Model file for the job. Use its own axes, mm. A direction names the side the tool comes from. Coordinates: 2 decimals unless noted, no trailing zeros. Order: outer loops, then holes, each group sorted by start corner. A loop starts at its lowest first (then second) coordinate and runs counter-clockwise, first axis right, second up. Notation, with made-up numbers: M 88.5,62 L 106.5,62 A29 ccw 106.5,89 Z; hole C 61.5,-38 d1. An arc over 180 degrees is marked long. Return JSON: item names as keys, results as strings.
```python
from build123d import *

# Parameters (mm, degrees)
F0_W     = 89
F0_H     = 23.8
F1_DEPTH = 3
F2_W     = 12
F2_H     = 6
F3_W     = 12
F3_H     = 6
F4_DEPTH = 9
F5_R     = 1.5
F6_DEPTH = 89.001
F7_R     = 1.5
F8_R     = 1.5
F9_DEPTH = 15


with BuildPart() as f1:
    # F0 (on Top) → F1 (new body)
    with BuildSketch(Plane.XY):
        Rectangle(F0_W, F0_H)
    extrude(amount=F1_DEPTH)

    # F2 (on face) + F3 (on face) → F4 (join)
    with BuildSketch(Plane.XY.offset(3)):
        with Locations((38.5, 8.9)):
            Rectangle(F2_W, F2_H)
    with BuildSketch(Plane.XY.offset(3)):
        with Locations((-38.5, 8.9)):
            Rectangle(F3_W, F3_H)
    extrude(amount=F4_DEPTH)

    # F5 (on face) → F6 (cut, through all)
    with BuildSketch(Plane(origin=(-44.5, 0, 0), x_dir=(0, -1, 0), z_dir=(-1, 0, 0))):
        with Locations((-8.9, 7.5)):
            Circle(F5_R)
    extrude(amount=-F6_DEPTH, mode=Mode.SUBTRACT)

    # F7 (on face) + F8 (on face) → F9 (cut)
    with BuildSketch(Plane.XY.offset(3)):
        with Locations((34.5, -6.9)):
            Circle(F7_R)
    with BuildSketch(Plane.XY.offset(3)):
        with Locations((-21.5, -6.9)):
            Circle(F8_R)
    extrude(amount=-F9_DEPTH, mode=Mode.SUBTRACT)


solid = f1.part
```
Item 1: Saw through at C-C (y = 8.9). Write the cut outline in (x, z), and give its area (3 significant figures).
Check result:
{"outline": "M -44.5,0 L 44.5,0 L 44.5,6 L 32.5,6 L 32.5,3 L -32.5,3 L -32.5,6 L -44.5,6 Z; M -44.5,9 L -32.5,9 L -32.5,12 L -44.5,12 Z; M 32.5,9 L 44.5,9 L 44.5,12 L 32.5,12 Z", "area": "411 mm2"}
Item 2: Saw through at D-D (x = -21.5). Write the cut outline in (y, z).
Check result:
{"outline": "M -11.9,0 L -8.4,0 L -8.4,3 L -11.9,3 Z; M -5.4,0 L 11.9,0 L 11.9,3 L -5.4,3 Z"}
Item 3: 3-axis set-ups, long thin cutter, end or side, ignore diameter. For faces 4 (the flat face through (38, 5.9, 7)), 5 (the flat face through (38, 9, 12)), 6 (the flat face through (32.5, 7.5, 8.4)): which of +Z, -Z, +X, -X, +Y, -Y reach the whole face in a straight line?
Check result:
{"face 4": "+Z, +X, -X, -Y", "face 5": "+Z, +X, -X, +Y, -Y", "face 6": "+Z, +Y, -Y"}
Item 4: Drop flat-ended pins along their axis: pin 1 Ø3 at (x, y) = (7, -3) entering from +Z; pin 2 Ø2.5 at (x, z) = (-36, 7) entering from -Y. Give the stop position or say it passes through.
Check result:
{"pin 1": "stops at z = 3", "pin 2": "stops at y = 5.9"}
Item 5: Saw through at B-B (x = 34.5). Write the cut outline in (y, z).
Check result:
{"outline": "M -11.9,0 L -8.4,0 L -8.4,3 L -11.9,3 Z; M -5.4,0 L 11.9,0 L 11.9,12 L 5.9,12 L 5.9,3 L -5.4,3 Z; hole C 8.9,7.5 d3"}
Item 6: Saw through at A-A (z = 5.25). Write the cut outline in (x, y), and give its area (3 significant figures).
Check result:
{"outline": "M -44.5,5.9 L -32.5,5.9 L -32.5,11.9 L -44.5,11.9 Z; M 32.5,5.9 L 44.5,5.9 L 44.5,11.9 L 32.5,11.9 Z", "area": "144 mm2"}
Item 7: Wall check: line 1 (X direction, y = -7, z = 1.5); line 2 (X direction, y = 10.5, z = 4); line 3 (Y direction, x = 34.5, z = 0.75). Give the ranges that are in metal, low to high.
Check result:
{"line 1": "x = -44.5 to -23, -20 to 33, 36 to 44.5", "line 2": "x = -44.5 to -32.5, 32.5 to 44.5", "line 3": "y = -11.9 to -8.4, -5.4 to 11.9"}
Item 8: Pull direction X, two halves, no side cores. Call faces 1 (the cylindrical face through (33.3, -7.8, 1.5)), 2 (the flat face through (44.5, 2, 2)), 3 (the flat face through (-39, 5.9, 7)): +X half, -X half, draft (parallel to the pull), parting line (faces both ways), or undercut.
Check result:
{"face 1": "undercut", "face 2": "+X half", "face 3": "draft"}
